Can you work these out from the drawing? Everything is in mm from the part's minimum corner. A direction names the side the tool comes from. Round coordinates to 2 decimals unless told otherwise and drop trailing zeros. Loops run counter-clockwise (first coordinate to the right, second up) from the corner with the lowest first, then second, coordinate; pieces in that order, holes last. Notation, with made-up numbers: M -35,48.25 L -9,48.25 A26 ccw -9,71.25 Z; hole C 46.5,76 d11. An arc over 180 degrees is marked long. Return JSON: item names as keys, results as strings. Group by question number.
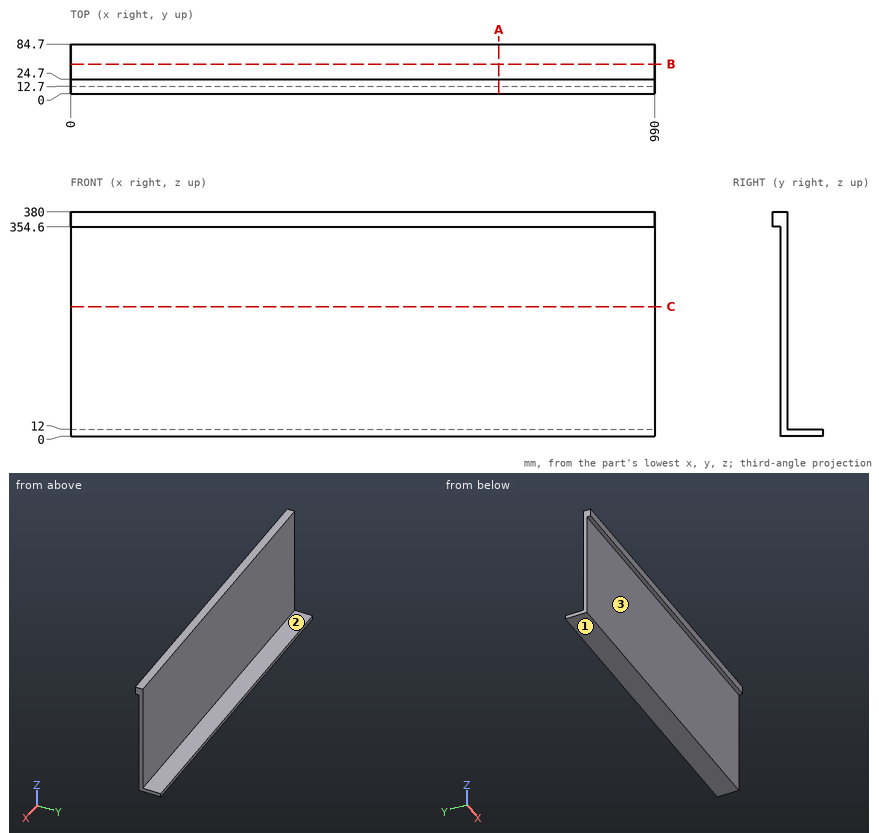
1. On a 3-axis mill with a long thin cutter (end or side, diameter ignored), from which of +Z, -Z, +X, -X, +Y, -Y can I reach the whole of each face in a straight line? I mean the marked faces 1, 2 and 3. Say none if no direction works.
2. I need wall thicknesses on probe 1 along Y at (x, z) = (483, 56.5); probe 2 along Z at (x, y) = (593.5, 28); probe 3 along Y at (x, z) = (328.5, 359). Which ranges of each line are inside material? Lowest first, please.
3. I'm going to push flat-ended pins straight in: pin 1 Ø10 at (x, z) = (125, 216) entering from -Y; pin 2 Ø14 at (x, y) = (637, 5) entering from -Z; pin 3 Ø2 at (x, y) = (408, 71) entering from +Z; pin 4 Ø4 at (y, z) = (12, 230) entering from -X. Where does each tip first touch, or does it pass through?
4. If we section it at C-C, the plane z = 219.5: Please give me the cut outline in (x, y).
5. If we section it at A-A, the plane x = 726: Please give me the cut outline in (y, z), then the cut area to 3 significant figures.
6. If we section it at B-B, the plane y = 50.5: Please give me the cut outline in (x, z).
Geometry results:
{
 "1": {"face 1": "-Z, +X, -X, +Y, -Y", "face 2": "+Z, +X, -X, +Y", "face 3": "-Z, +X, -X, -Y"},
 "2": {"probe 1": "12.7 to 24.7", "probe 2": "0 to 12", "probe 3": "0 to 24.7"},
 "3": {"pin 1": "y = 12.7", "pin 2": "z = 354.6", "pin 3": "z = 12", "pin 4": "x = 0"},
 "4": {"outline": "M 0,12.7 L 990,12.7 L 990,24.7 L 0,24.7 Z"},
 "5": {"outline": "M 0,354.6 L 12.7,354.6 L 12.7,0 L 84.7,0 L 84.7,12 L 24.7,12 L 24.7,380 L 0,380 Z", "area": "5,600 mm^2"},
 "6": {"outline": "M 0,0 L 990,0 L 990,12 L 0,12 Z"}
}
